For this review, take the finished solid that the model builds, in its own axes (mm). Round coordinates to 2 decimals unless told otherwise and drop trailing zeros. Write each loop counter-clockwise with the first axis right and the second up, starting at its lowest first coordinate (ties: lowest second). Pieces come first, ordered by that corner, then holes. Notation, with made-up numbers: (-22.5, -23.5) -> (14.5, -23.5) arc R34 ccw to (14.5, 12.5) -> close; hole circle Ø2 at (16, 34.25). An arc over 180 degrees is marked (long way). Write each question's results on one line, items separated by ' | '. Start each with the question number.
Item 1: Add section B-B (z = -25). State the section outline as (x, y) points.
Item 2: Add section A-A (y = 0). State the section outline as (x, z) points, plus the area to 3 significant figures.
Item 3: Clearance check with flat-ended pins moving along their axes: pin 1 (5 mm diameter, centred on y = -8, z = -38.5, fed in from +X); pin 2 (8 mm diameter, centred on x = -21.5, z = -38.5, fed in from +Y); pin 3 (9.5 mm diameter, centred on x = 0, y = 0, fed in from -Z). State where each tip first meets the part, or that it passes through.
Item 4: The part is to be moulded in two halves that separate along Y. For faces 1 (the cylindrical face through (14.434, 16.18, 5.07)), 2 (the flat face through (-39, -30, -25)), 3 (the flat face through (0, -25, -30)), say which applies: +Y half, -Y half, draft (parallel to the pull), parting line (faces both ways), or undercut.
Item 5: Add section D-D (z = -40.5). State the section outline as (x, y) points, plus the area to 3 significant figures.
Item 6: Add section C-C (y = -24). State the section outline as (x, z) points.
Item 7: To check wall thickness, follow line 1 along Y through (x, z) = (-72, -40.5); line 2 along Z through (x, y) = (-76.75, 15.5); line 3 along Y through (x, z) = (-75, -9). State the ranges of each line that lie inside material, in increasing order.
Autodesk Fusion 360 part; units mm, degrees
sketch "Sketch1" plane through (0, 0, 0) normal (0, 0, 1) x (1, 0, 0)
  circle A0 centre (0, 0) radius 30
  dimension "d1" = 60
extrude "Extrude1" add sketch "Sketch1" along normal blind 10
sketch "Sketch2" plane through (0, 0, 10) normal (0, 0, 1) x (1, 0, 0)
  circle A0 centre (0, 0) radius 30
  line L0 (0, -30) -> (-80, -30)
  line L1 (-80, -30) -> (-80, -20)
  line L2 (-80, -20) -> (0, -20)
  line L3 (0, -20) -> (0, -30)
  dimension "d4" = 80
  dimension "d5" = 10
extrude "Extrude2" add sketch "Sketch2" against normal blind 70 contours A0 L0 L1 L2 | A0 L2 L3 picked at (-1.3972, -26.5686)
sketch "Sketch3" plane through (-80, 0, 0) normal (-1, 0, 0) x (0, 0, 1)
  line L0 (10, -30) -> (10, -20)
  line L1 (10, -20) -> (-60, -20)
  line L2 (-60, -20) -> (-60, -30)
  line L3 (-60, -30) -> (10, -30)
  circle A0 centre (-25, 0) radius 30
  line L4 (-25, -30) -> (-25, 0) construction
  dimension "d8" = 60
extrude "Extrude3" add sketch "Sketch3" against normal blind 10 contours L1 A0 picked at (-32.7403, 15.1228)
sketch "Sketch4" plane through (0, 0, 0) normal (0, 0, -1) x (-1, 0, 0)
  line L0 (0, -30) -> (0, -20)
  line L1 (0, -20) -> (22.3607, -20)
  arc A0 (22.3607, -20) -> (0, -30) centre (0, 0) ccw
  line L2 (15.5, -15.5) -> (-15.5, -15.5)
  line L3 (-15.5, -15.5) -> (-15.5, 15.5)
  line L4 (-15.5, 15.5) -> (15.5, 15.5)
  line L5 (15.5, 15.5) -> (15.5, -15.5)
  line L6 (15.5, -15.5) -> (-15.5, 15.5) construction
  line L7 (-15.5, -15.5) -> (15.5, 15.5) construction
  dimension "d11" = 31
  dimension "d12" = 31
hole "Hole1" at (-15.5, 15.5, 0) at (15.5, 15.5, 0) at (15.5, -15.5, 0) at (-15.5, -15.5, 0) direction (0, 0, 1) diameter 2.529 depth 10 tip angle 118
hole "Hole2" at (0, 0, 0) direction (0, 0, 1) diameter 6 depth 10 tip angle 118
sketch "Sketch5" plane through (-80, 0, 0) normal (-1, 0, 0) x (0, 0, 1)
  line L0 (10, -30) -> (10, -20)
  line L1 (10, -20) -> (-2.6393, -20)
  arc A0 (-2.6393, -20) -> (-47.3607, -20) centre (-25, 0) ccw
  line L2 (-47.3607, -20) -> (-60, -20)
  line L3 (-60, -20) -> (-60, -30)
  line L4 (-60, -30) -> (10, -30)
  line L5 (-40.5, 15.5) -> (-9.5, 15.5)
  line L6 (-9.5, 15.5) -> (-9.5, -15.5)
  line L7 (-9.5, -15.5) -> (-40.5, -15.5)
  line L8 (-40.5, -15.5) -> (-40.5, 15.5)
  line L9 (-40.5, 15.5) -> (-9.5, -15.5) construction
  line L10 (-9.5, 15.5) -> (-40.5, -15.5) construction
  point P0 (-25, 0)
  dimension "d19" = 31
  dimension "d20" = 31
hole "Hole3" at (-80, 15.5, -40.5) at (-80, 15.5, -9.5) at (-80, -15.5, -40.5) at (-80, -15.5, -9.5) direction (1, 0, 0) diameter 3.332 depth 40 tip angle 118
hole "Hole4" at (-80, 0, -25) direction (1, 0, 0) diameter 6 depth 40 tip angle 118
Responses:
1) outline: (-80, -30) -> (0, -30) -> (0, -20) -> (-70, -20) -> (-70, -3) -> (-80, -3) -> close; (-80, 3) -> (-70, 3) -> (-70, 30) -> (-80, 30) -> close
2) outline: (-80, -55) -> (-70, -55) -> (-70, -28) -> (-80, -28) -> close; (-80, -22) -> (-70, -22) -> (-70, 5) -> (-80, 5) -> close; (-30, 0) -> (-3, 0) -> (-3, 10) -> (-30, 10) -> close; (3, 0) -> (30, 0) -> (30, 10) -> (3, 10) -> close | area: 1,080 mm^2
3) pin 1: stops at x = -70 | pin 2: stops at y = -20 | pin 3: stops at z = 0
4) face 1: undercut | face 2: -Y half | face 3: draft
5) outline: (-80, -30) -> (0, -30) -> (0, -20) -> (-70, -20) -> (-70, -17.17) -> (-80, -17.17) -> close; (-80, -13.83) -> (-70, -13.83) -> (-70, 13.83) -> (-80, 13.83) -> close; (-80, 17.17) -> (-70, 17.17) -> (-70, 25.69) -> (-80, 25.69) -> close | area: 1,190 mm^2
6) outline: (-80, -60) -> (0, -60) -> (0, 0) -> (18, 0) -> (18, 10) -> (-80, 10) -> close
7) line 1: y = -30 to -17.17, -13.83 to 13.83, 17.17 to 25.69 | line 2: z = -50.69 to -42.17, -38.83 to -11.17, -7.83 to 0.69 | line 3: y = -30 to -17.09, -13.91 to 13.91, 17.09 to 25.38
